Design review of the part built by this model. Coordinates are the model's own, in mm. Coordinates: 2 decimals unless noted, no trailing zeros. Loops run counter-clockwise (first coordinate to the right, second up) from the corner with the lowest first, then second, coordinate; pieces in that order, holes last. Notation, with made-up numbers: (-16.75, 86.5) - (41.25, 86.5) arc R17 ccw to (41.25, 112.5) - close; hole circle Ø8 at (33.25, -20). An arc over 180 degrees is marked (long way). One line per question, with ' | ' between items.
from build123d import *

# Parameters (mm, degrees)
BOSS_EXTRUDE1_DEPTH = 4
TAP1_D              = 4.134


with BuildPart() as part:
    # Sketch1 → Boss-Extrude1 (new body)
    with BuildSketch(Plane(origin=(0, 0, 0), x_dir=(0, 0, -1), z_dir=(1, 0, 0))):
        Polygon((0, 4.618802154), (-4, 2.309401077), (-4, -2.309401077), (0, -4.618802154), (4, -2.309401077), (4, 2.309401077), align=None)
    extrude(amount=-BOSS_EXTRUDE1_DEPTH)

    # Sketch2 → Cut-Revolve1 (revolve, cut)
    with BuildSketch(Plane.XY):
        Polygon((-4, 4), (-3.64273441, 4.618802154), (-4, 4.618802154), align=None)
    revolve(axis=Axis((-2.23854625, 0, 0), (1, 0, 0)), mode=Mode.SUBTRACT)

    # Tap1 (through all)
    with Locations(Plane.ZY.offset(4)):
        with Locations((0, 0)):
            Hole(TAP1_D / 2)


solid = part.part
Q1. To check wall thickness, follow line 1 along Y through (x, z) = (-1.8, -0.5); line 2 along Y through (x, z) = (-1.4, 1.5); line 3 along Z through (x, y) = (-2.7, -0.5). State the ranges of each line that lie inside material, in increasing order.
Returned:
line 1: y = -4.33 to -2.01, 2.01 to 4.33 | line 2: y = -3.75 to -1.42, 1.42 to 3.75 | line 3: z = -4 to -2.01, 2.01 to 4
Q2. Take a section at A-A (x = -3.05). Give the boundary of the cut face in (y, z).
Returned:
outline: (-4.62, 0) - (-2.31, -4) - (2.31, -4) - (4.62, 0) - (2.31, 4) - (-2.31, 4) - close; hole circle Ø4.13 at (0, 0)
Q3. For pin 1 (2 mm diameter, centred on y = 2, z = -0.5, fed in from +X), flat-tipped, find the tip position at first contact; note if it passes through.
Returned:
pin 1: stops at x = 0
